```python
from build123d import *

# Parameters (mm, degrees)
F0_W     = 500
F0_H     = 175
F1_DEPTH = 10
F5_R     = 14.75
F5_R_2   = 12.4064380464
F7_DEPTH = 25
F3_R     = 14.75
F3_R_2   = 12
F8_DEPTH = 25
F6_R     = 14
F9_DEPTH = 25


# Not quite as in the source:
# - a feature names something its author has since deleted; it is built from what else it names


with BuildPart() as f1:
    # F0 (on Front) → F1 (new body)
    with BuildSketch(Plane.XZ):
        with Locations((250, 87.5)):
            Rectangle(F0_W, F0_H)
    extrude(amount=F1_DEPTH)

    # F5 (on face) → F7 (cut)
    with BuildSketch(Plane.XZ.offset(10)):
        with Locations((354.5, 106.75)):
            Circle(F5_R)
        with Locations((385.5, 127)):
            Circle(F5_R)
        with Locations((422, 127)):
            Circle(F5_R)
        with Locations((422, 87.5)):
            Circle(F5_R)
        with Locations((385.5, 87.5)):
            Circle(F5_R)
        with Locations((354.5, 67.25)):
            Circle(F5_R)
        with Locations((291.5, 87.5)):
            Circle(F5_R_2)
    extrude(amount=-F7_DEPTH, mode=Mode.SUBTRACT)

    # F3 (on face) → F8 (cut)
    with BuildSketch(Plane.XZ.offset(10)):
        with Locations((177, 126.3350188136)):
            Circle(F3_R)
        with Locations((212.5, 120.3350188136)):
            Circle(F3_R)
        with Locations((206, 81.8350188136)):
            Circle(F3_R)
        with Locations((170, 87.8350188136)):
            Circle(F3_R)
        with Locations((137, 73.8350188136)):
            Circle(F3_R)
        with Locations((144, 112.3350188136)):
            Circle(F3_R)
        with Locations((78, 87.5)):
            Circle(F3_R_2)
    extrude(amount=-F8_DEPTH, mode=Mode.SUBTRACT)

    # F6 (on face) → F9 (cut)
    with BuildSketch(Plane.XZ.offset(10)):
        with Locations((263.5, 145)):
            Circle(F6_R)
        with Locations((50, 145)):
            Circle(F6_R)
        with Locations((90, 145)):
            Circle(F6_R)
        with Locations((303.5, 145)):
            Circle(F6_R)
        with Locations((460, 145)):
            Circle(F6_R)
    extrude(amount=-F9_DEPTH, mode=Mode.SUBTRACT)


solid = f1.part
```
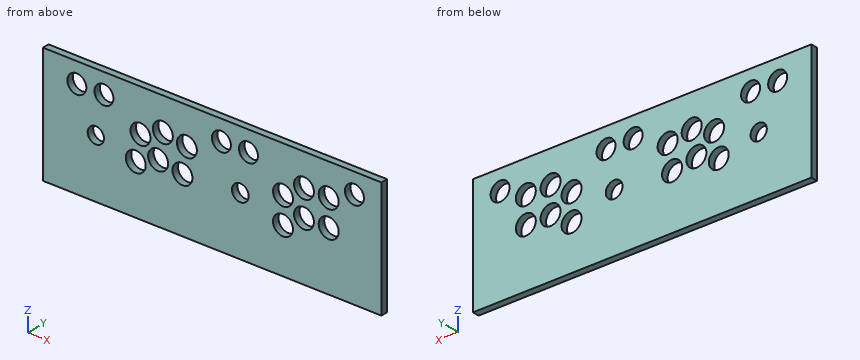
Design review of the part built by this model. Coordinates are the model's own, in mm. Round coordinates to 2 decimals unless told otherwise and drop trailing zeros. Write each loop counter-clockwise with the first axis right and the second up, starting at its lowest first coordinate (ties: lowest second). Pieces come first, ordered by that corner, then holes.
Item 1: We need section B-B on y = -2.5. State how many separate pieces and enclosed holes the cut face has, and give its area (3 significant figures).
Item 2: We need section C-C on x = 137. Write out the cut boundary in (y, z), and give its area (3 significant figures).
Item 3: For probe 1 along Z at (x, y) = (137, -6.75); probe 2 along Z at (x, y) = (210.5, -5.75); probe 3 along X at (y, z) = (-8.75, 103), list the stretches that pass through material, from the lowest coordinate up.
Item 4: We need section A-A on x = 385.5. Write out the cut boundary in (y, z).
Returned:
1. separate pieces: 1
1. enclosed holes: 19
1. area: 75,300 mm2
2. outline: (-10, 0) - (0, 0) - (0, 59.09) - (-10, 59.09) - close; (-10, 88.59) - (0, 88.59) - (0, 99.35) - (-10, 99.35) - close; (-10, 125.32) - (0, 125.32) - (0, 175) - (-10, 175) - close
2. area: 1,200 mm2
3. probe 1: z = 0 to 59.09, 88.59 to 99.35, 125.32 to 175
3. probe 2: z = 0 to 67.79, 95.88 to 105.72, 134.95 to 175
3. probe 3: x = 0 to 132.58, 155.42 to 340.23, 368.77 to 500
4. outline: (-10, 0) - (0, 0) - (0, 72.75) - (-10, 72.75) - close; (-10, 102.25) - (0, 102.25) - (0, 112.25) - (-10, 112.25) - close; (-10, 141.75) - (0, 141.75) - (0, 175) - (-10, 175) - close
